Input: part model. Units: mm. Frame: model coordinates. A direction names the side the tool comes from. Give positions to 0.01 mm unless a question says otherwise; leave off trailing zeros. Order: outer loops, then holes, each group sorted by start corner. A loop starts at its lowest first (then second) coordinate and runs counter-clockwise, first axis right, second up. Notation, with made-up numbers: (-22, 46) - (37, 46) arc R34 cw to (37, 76) - close; hole circle Ø1 at (3, 55). An arc over 180 degrees is marked (long way). Use a Markdown table: item, result.
from build123d import *

# Parameters (mm, degrees)
BOSS_EXTRUDE1_DEPTH      = 2.5
BOSS_EXTRUDE1_DEPTH_BACK = 2.5
SKETCH1_W                = 7.31
SKETCH1_H                = 8.1
SKETCH2_R                = 0.4
BOSS_EXTRUDE2_DEPTH      = 0.8
FILLET1_R                = 0.4
SKETCH3_R                = 0.35
BOSS_EXTRUDE3_DEPTH      = 0.35
LPATTERN1_COUNT          = 2
LPATTERN1_PITCH          = 2.2
LPATTERN2_COUNT          = 2
LPATTERN2_PITCH          = 2.2
FILLET2_R                = 0.2
SKETCH4_R                = 2.975
BOSS_EXTRUDE4_DEPTH      = 0.3
SKETCH5_R                = 2.36
BOSS_EXTRUDE5_DEPTH      = 5.5
SHELL1_START             = -3.255
SHELL1_OUTLINE_W         = 7.3
SHELL1_OUTLINE_H         = 4.2
SHELL1_DEPTH             = 6.51
SHELL1_START_2           = 3.255
SHELL1_2_OUTLINE_R       = 1.96
SHELL1_2_DEPTH           = 6.2
SHELL1_3_OUTLINE_R       = 1.96
SHELL1_3_DEPTH           = 0.3


# Read off the part's stored shape, not the designer's step: Shell1
with BuildPart() as part:
    # Sketch1 → Boss-Extrude1 (new, two sides: drawn at the far end of the back side and taken through both)
    with BuildSketch(Plane.XY.offset(-BOSS_EXTRUDE1_DEPTH_BACK)):
        Rectangle(SKETCH1_W, SKETCH1_H)
    extrude(amount=BOSS_EXTRUDE1_DEPTH + BOSS_EXTRUDE1_DEPTH_BACK)

    # Sketch2 → Boss-Extrude2 (add)
    with BuildSketch(Plane.ZY.offset(3.655)):
        with Locations(Location((2.1, 3.65, 0), (0, 0, 90))):
            Circle(SKETCH2_R)
        with Locations(Location((2.1, -3.65, 0), (0, 0, 90))):
            Circle(SKETCH2_R)
        with Locations(Location((-2.1, -3.65, 0), (0, 0, 270))):
            Circle(SKETCH2_R)
        with Locations(Location((-2.1, 3.65, 0), (0, 0, 90))):
            Circle(SKETCH2_R)
    extrude(amount=BOSS_EXTRUDE2_DEPTH)

    # Fillet1
    fillet1_edges = [part.edges().sort_by_distance(p)[0] for p in [
        (-4.455, 3.25, 2.1),
        (-4.455, -4.05, 2.1),
        (-4.455, -3.25, -2.1),
        (-4.455, 3.25, -2.1),
    ]]
    fillet(fillet1_edges, radius=FILLET1_R)

    # Sketch3 → Boss-Extrude3 (add, symmetric)
    with BuildSketch(Plane(origin=(0, 0, 0), x_dir=(1, 0, 0), z_dir=(0, 1, 0))):
        Polygon((-3.655, 1.55), (-4.455, 1.55), (-4.455, 0.85), (-6.755, 0.85), (-6.755, -0.85), (-4.455, -0.85), (-4.455, -1.55), (-3.655, -1.55), align=None)
        with Locations(Location((-5.605, 0, 0), (0, 0, 270))):
            Circle(SKETCH3_R, mode=Mode.SUBTRACT)
    boss_extrude3 = extrude(amount=BOSS_EXTRUDE3_DEPTH, both=True)

    # LPattern1: Boss-Extrude3 ×2
    with Locations(*[(0, -i * LPATTERN1_PITCH, 0) for i in range(1, LPATTERN1_COUNT)]):
        add(boss_extrude3)

    # LPattern2: Boss-Extrude3 ×2
    with Locations(*[(0, i * LPATTERN2_PITCH, 0) for i in range(1, LPATTERN2_COUNT)]):
        add(boss_extrude3)

    # Fillet2
    fillet2_edges = [part.edges().sort_by_distance(p)[0] for p in [
        (-6.755, 2.2, -0.85),
        (-4.455, 2.2, -0.85),
        (-4.455, 2.2, -1.55),
        (-4.455, 2.2, 1.55),
        (-4.455, 2.2, 0.85),
        (-6.755, 2.2, 0.85),
        (-6.755, 0, -0.85),
        (-4.455, 0, -0.85),
        (-4.455, 0, -1.55),
        (-4.455, 0, 1.55),
        (-4.455, 0, 0.85),
        (-6.755, 0, 0.85),
        (-6.755, -2.2, -0.85),
        (-4.455, -2.2, -0.85),
        (-4.455, -2.2, -1.55),
        (-4.455, -2.2, 1.55),
        (-4.455, -2.2, 0.85),
        (-6.755, -2.2, 0.85),
    ]]
    fillet(fillet2_edges, radius=FILLET2_R)

    # Sketch4 → Boss-Extrude4 (add)
    with BuildSketch(Plane(origin=(3.655, 0, 0), x_dir=(0, 0, -1), z_dir=(1, 0, 0))):
        with Locations(Location((0, 0, 0), (0, 0, 212.824368373))):
            Circle(SKETCH4_R)
    extrude(amount=BOSS_EXTRUDE4_DEPTH)

    # Sketch5 → Boss-Extrude5 (add)
    with BuildSketch(Plane(origin=(3.955, 0, 0), x_dir=(0, 0, -1), z_dir=(1, 0, 0))):
        with Locations(Location((0, 0, 0), (0, 0, 90))):
            Circle(SKETCH5_R)
    extrude(amount=BOSS_EXTRUDE5_DEPTH)

    # Shell1 outline → Shell1 (cut)
    with BuildSketch(Plane.YZ.offset(SHELL1_START)):
        Rectangle(SHELL1_OUTLINE_W, SHELL1_OUTLINE_H)
    extrude(amount=SHELL1_DEPTH, mode=Mode.SUBTRACT)

    # Shell1 2 outline → Shell1 2 (cut)
    with BuildSketch(Plane.YZ.offset(SHELL1_START_2)):
        Circle(SHELL1_2_OUTLINE_R)
    extrude(amount=SHELL1_2_DEPTH, mode=Mode.SUBTRACT)

    # Shell1 3 outline → Shell1 3 (cut)
    with BuildSketch(Plane.YZ.offset(SHELL1_START_2)):
        with BuildLine():
            ThreePointArc((-1.490176164, 2.1), (-2.575, 0), (-1.490176164, -2.1))
            Line((-1.490176164, -2.1), (1.490176164, -2.1))
            ThreePointArc((1.490176164, -2.1), (2.575, 0), (1.490176164, 2.1))
            Line((1.490176164, 2.1), (-1.490176164, 2.1))
        make_face()
        Circle(SHELL1_3_OUTLINE_R, mode=Mode.SUBTRACT)
    extrude(amount=SHELL1_3_DEPTH, mode=Mode.SUBTRACT)


solid = part.part
1. Mould query, pull axis Y, two halves, no side actions, for faces 1 (the face through (3.255, 3, 0)), 2 (the face through (0, -4.05, 0)), 3 (the face through (6.666, 1.089, -2.094)). Classes: pulls with the +Y half, pulls with the -Y half, needs draft (parallel to the pull), parting line crosses it, or undercut.
Response:
| item | result |
|---|---|
| face 1 | undercut |
| face 2 | pulls with the -Y half |
| face 3 | parting line crosses it |
2. Section query B-B (z = 0). State how many separate pieces and enclosed holes the cut face has, then the cut area to 3 significant figures.
Response:
| item | result |
|---|---|
| separate pieces | 4 |
| enclosed holes | 0 |
| area | 19.8 mm^2 |
3. Material intervals for line 1 along X through (y, z) = (2.3, 0) (3 decimals); line 2 along Z through (x, y) = (-2.75, 2); line 3 along X through (y, z) = (3, -0.8) (3 decimals), sorted ascending.
Response:
| item | result |
|---|---|
| line 1 | x = -6.755 to -5.955, -5.255 to -3.255, 3.555 to 9.455 |
| line 2 | z = -2.5 to -2.1, 2.1 to 2.5 |
| line 3 | x = -3.655 to -3.255, 3.255 to 3.655 |
4. Pin query (flat end, axial travel): pin 1 (0.6 mm diameter, centred on x = -5.5, y = 0, fed in from -Z); pin 2 (1.5 mm diameter, centred on x = 7, y = 0, fed in from -Z); pin 3 (1.6 mm diameter, centred on x = -4.5, z = -0.5, fed in from -Y). Return the tip coordinate at first contact, or that it passes through.
Response:
| item | result |
|---|---|
| pin 1 | stops at z = -0.85 |
| pin 2 | stops at z = -2.36 |
| pin 3 | stops at y = -2.55 |
5. Section query A-A (x = -0.5). Return loops of the section in (y, z), then the cut area to 3 significant figures.
Response:
| item | result |
|---|---|
| outline | (-4.05, -2.5) - (4.05, -2.5) - (4.05, 2.5) - (-4.05, 2.5) - close; hole (-3.65, -2.1) - (3.65, -2.1) - (3.65, 2.1) - (-3.65, 2.1) - close |
| area | 9.84 mm^2 |
6. Set-up query: faces 4 (the face through (0, -3.65, 0)), 5 (the face through (-5, 1.85, 0)), 6 (the face through (0, 0, -2.5)). Return all of +Z, -Z, +X, -X, +Y, -Y with unobstructed straight access to the full face (end or side cutting, diameter ignored); none if empty.
Response:
| item | result |
|---|---|
| face 4 | none |
| face 5 | +Z, -Z, -X |
| face 6 | -Z, -X, +Y, -Y |
7. Section query C-C (y = -1). Return loops of the section in (x, z) (3 decimals), then the cut area to 3 significant figures.
Response:
| item | result |
|---|---|
| outline | (-3.655, -2.5) - (3.655, -2.5) - (3.655, -2.802) - (3.955, -2.802) - (3.955, -2.138) - (9.455, -2.138) - (9.455, -1.686) - (3.555, -1.686) - (3.555, -2.1) - (-3.255, -2.1) - (-3.255, 2.1) - (3.555, 2.1) - (3.555, 1.686) - (9.455, 1.686) - (9.455, 2.138) - (3.955, 2.138) - (3.955, 2.802) - (3.655, 2.802) - (3.655, 2.5) - (-3.655, 2.5) - close |
| area | 13.3 mm^2 |
